```python
from build123d import *

# Parameters (mm, degrees)
SKETCH2_W           = 220
SKETCH2_H           = 180
BOSS_EXTRUDE1_DEPTH = 4.5
CHAMFER1_SIZE       = 75
CHAMFER1_SIZE2      = 62.932472338
SKETCH3_R           = 8
CUT_EXTRUDE1_DEPTH  = 143.197925442
SKETCH4_W           = 20
SKETCH4_H           = 4.4
CUT_EXTRUDE2_DEPTH  = 143.197925442


with BuildPart() as part:
    # Sketch2 → Boss-Extrude1 (new body)
    with BuildSketch(Plane(origin=(0, 0, 0), x_dir=(1, 0, 0), z_dir=(0, 1, 0))):
        Rectangle(SKETCH2_W, SKETCH2_H)
    extrude(amount=BOSS_EXTRUDE1_DEPTH)

    # Chamfer1
    chamfer1_edges = [part.edges().sort_by_distance(p)[0] for p in [
        (110, 2.25, 90),
        (-110, 2.25, 90),
    ]]
    chamfer1_side = [part.faces().sort_by_distance(p)[0] for p in [
        (0, 2.25, 90),
    ]]
    chamfer(chamfer1_edges, length=CHAMFER1_SIZE, length2=CHAMFER1_SIZE2, reference=chamfer1_side[0])

    # Sketch3 → Cut-Extrude1 (cut, through all)
    with BuildSketch(Plane(origin=(0, 4.5, 0), x_dir=(1, 0, 0), z_dir=(0, 1, 0))):
        with Locations(Location((0, -40, 0), (0, 0, 270))):
            Circle(SKETCH3_R)
        with Locations(Location((40.6, 40, 0), (0, 0, 270))):
            Circle(SKETCH3_R)
    extrude(amount=-CUT_EXTRUDE1_DEPTH, mode=Mode.SUBTRACT)

    # Sketch4 → Cut-Extrude2 (cut, through all)
    with BuildSketch(Plane.XZ):
        with Locations((100, -87.8)):
            Rectangle(SKETCH4_W, SKETCH4_H)
        with Locations((60, -87.8)):
            Rectangle(SKETCH4_W, SKETCH4_H)
        with Locations((20, -87.8)):
            Rectangle(SKETCH4_W, SKETCH4_H)
        with Locations((-20, -87.8)):
            Rectangle(SKETCH4_W, SKETCH4_H)
        with Locations((-60, -87.8)):
            Rectangle(SKETCH4_W, SKETCH4_H)
        with Locations((-100, -87.8)):
            Rectangle(SKETCH4_W, SKETCH4_H)
    extrude(amount=-CUT_EXTRUDE2_DEPTH, mode=Mode.SUBTRACT)


solid = part.part
```
The listing builds one solid part. Answer for the finished solid, in the listing's coordinates (mm). A direction names the side the tool comes from. Coordinates: 2 decimals unless noted, no trailing zeros. Write each loop counter-clockwise with the first axis right and the second up, starting at its lowest first coordinate (ties: lowest second). Pieces come first, ordered by that corner, then holes. Notation, with made-up numbers: (1.5, 3) -> (34.5, 3) arc R22 ccw to (34.5, 42) -> close; hole circle Ø3 at (-12.75, 50). An arc over 180 degrees is marked (long way). Write each question's results on one line, items separated by ' | '. Start each with the question number.
1) A cutting plane is placed at A-A (x = 0). Determine the outline of the cut face in (y, z).
2) Flat-ended cylindrical pins translate along their axes: pin 1 Ø1.3 at (y, z) = (1, -87.5) entering from -X; pin 2 Ø13 at (x, z) = (0, 40) entering from +Y; pin 3 Ø2 at (y, z) = (0.5, 58.5) entering from -X; pin 4 Ø1.3 at (x, y) = (97, 1.5) entering from -Z. Find the tip coordinate at first contact, or state that the pin passes through.
3) A cutting plane is placed at C-C (y = 2.8). Determine the outline of the cut face in (x, z), then the cut area to 4 significant figures.
4) A cutting plane is placed at D-D (x = 60.5). Determine the outline of the cut face in (y, z).
5) A tool of negligible diameter and unlimited length cuts with its end or side. For faces 1 (the flat face through (90, 2, -88)), 2 (the flat face through (-40, 2, -90)), 3 (the flat face through (-30, 2, -88)), 4 (the flat face through (-100, 2, -85.6)), 5 (the flat face through (110, 2, -28)), from which of +Z, -Z, +X, -X, +Y, -Y can it reach the whole face along a straight path? Write none if from no direction.
6) A cutting plane is placed at B-B (z = -40). Determine the outline of the cut face in (x, y).
7) Straight lines are drawn through the part: probe 1 along X at (y, z) = (2.1, 40); probe 2 along X at (y, z) = (1.75, -40); probe 3 along Z at (x, y) = (26.5, 1.65). For each, find the intervals that lie inside material, in ascending order.
Values follow:
1) outline: (0, -90) -> (4.5, -90) -> (4.5, 32) -> (0, 32) -> close; (0, 48) -> (4.5, 48) -> (4.5, 90) -> (0, 90) -> close
2) pin 1: x = -90 | pin 2: through | pin 3: x = -73.73 | pin 4: z = -85.6
3) outline: (-110, -85.6) -> (-90, -85.6) -> (-90, -90) -> (-70, -90) -> (-70, -85.6) -> (-50, -85.6) -> (-50, -90) -> (-30, -90) -> (-30, -85.6) -> (-10, -85.6) -> (-10, -90) -> (10, -90) -> (10, -85.6) -> (30, -85.6) -> (30, -90) -> (50, -90) -> (50, -85.6) -> (70, -85.6) -> (70, -90) -> (90, -90) -> (90, -85.6) -> (110, -85.6) -> (110, 27.07) -> (35, 90) -> (-35, 90) -> (-110, 27.07) -> close; hole circle Ø16 at (0, 40); hole circle Ø16 at (40.6, -40) | area: 33,950 mm²
4) outline: (0, -85.6) -> (4.5, -85.6) -> (4.5, 68.6) -> (0, 68.6) -> close
5) face 1: -Z, +X, +Y, -Y | face 2: -Z, +X, -X, +Y, -Y | face 3: -Z, +Y, -Y | face 4: -Z, -X, +Y, -Y | face 5: +Z, -Z, +X, +Y, -Y
6) outline: (-110, 0) -> (32.6, 0) -> (32.6, 4.5) -> (-110, 4.5) -> close; (48.6, 0) -> (110, 0) -> (110, 4.5) -> (48.6, 4.5) -> close
7) probe 1: -94.59 to -8, 8 to 94.59 | probe 2: -110 to 32.6, 48.6 to 110 | probe 3: -85.6 to 90
